```python
from build123d import *
from build123d.topology import SkipClean

# Parameters (mm, degrees)
BOSS_EXTRUDE1_START   = -10
BOSS_EXTRUDE1_DEPTH   = 40
SKETCH1_W             = 30
SKETCH1_H             = 10
BOSS_EXTRUDE1_2_DEPTH = 40
EXTRUDE_THIN1_DEPTH   = 60
BOSS_EXTRUDE2_DEPTH   = 30
BOSS_EXTRUDE3_START   = -10
BOSS_EXTRUDE3_DEPTH   = 10
FILLET2_R             = 10
BOSS_EXTRUDE4_DEPTH   = 5
CUT_EXTRUDE1_DEPTH    = 124.693168817
BOSS_EXTRUDE6_DEPTH   = 10


with BuildPart() as part:
    # Sketch1 → Boss-Extrude1 (new body)
    with BuildSketch(Plane.XY.offset(BOSS_EXTRUDE1_START)):
        with BuildLine():
            Line((60, 10), (38.729833462, 10))
            ThreePointArc((38.729833462, 10), (39.681187851, 5.040171699), (40, 0))
            Line((40, 0), (60, 0))
            Line((60, 0), (60, 10))
        make_face()
    extrude(amount=-BOSS_EXTRUDE1_DEPTH)



with BuildPart() as body_2:
    # Sketch1 → Boss-Extrude1 2 (new body)
    with BuildSketch(Plane.XY.offset(BOSS_EXTRUDE1_START)):
        with Locations((-45, 5)):
            Rectangle(SKETCH1_W, SKETCH1_H)
    extrude(amount=-BOSS_EXTRUDE1_2_DEPTH)


with BuildPart() as part_1:
    add(part.part)

    add(body_2.part)  # Extrude-Thin1 merges body 2
    # Sketch1<3> → Extrude-Thin1 (add)
    with BuildSketch(Plane.XY):
        with BuildLine():
            ThreePointArc((30, 0), (0, 30), (-30, 0))
            Line((-30, 0), (-40, 0))
            ThreePointArc((-40, 0), (0, 40), (40, 0))
            Line((40, 0), (30, 0))
        make_face()
    extrude(amount=-EXTRUDE_THIN1_DEPTH)



with BuildPart() as body_2_2:
    # Sketch2 → Boss-Extrude2 (new body)
    with BuildSketch(Plane(origin=(0, 0, -60), x_dir=(-1, 0, 0), z_dir=(0, 0, -1))):
        with BuildLine():
            ThreePointArc((-25, 100), (-17.67766953, 82.32233047), (0, 75))
            Line((0, 75), (0, 85))
            ThreePointArc((0, 85), (-10.606601718, 89.393398282), (-15, 100))
            Line((-15, 100), (-25, 100))
        make_face()
        with BuildLine():
            Line((0, 85), (0, 75))
            ThreePointArc((0, 75), (17.67766953, 82.32233047), (25, 100))
            Line((25, 100), (15, 100))
            ThreePointArc((15, 100), (10.606601718, 89.393398282), (0, 85))
        make_face()
    extrude(amount=-BOSS_EXTRUDE2_DEPTH)


with BuildPart() as part_2:
    add(part_1.part)

    add(body_2_2.part)  # Boss-Extrude3 merges body 2 2
    # Sketch2<5> → Boss-Extrude3 (add)
    with BuildSketch(Plane(origin=(0, 0, -60), x_dir=(-1, 0, 0), z_dir=(0, 0, -1)).offset(BOSS_EXTRUDE3_START)):
        with BuildLine():
            ThreePointArc((-38.239608802, 11.73594132), (-23.775642443, 32.167045659), (0, 40))
            Line((0, 40), (0, 75))
            ThreePointArc((0, 75), (-17.67766953, 82.32233047), (-25, 100))
            Line((-25, 100), (-38.239608802, 11.73594132))
        make_face()
        with BuildLine():
            Line((0, 75), (0, 40))
            ThreePointArc((0, 40), (23.775642443, 32.167045659), (38.239608802, 11.73594132))
            Line((38.239608802, 11.73594132), (25, 100))
            ThreePointArc((25, 100), (17.67766953, 82.32233047), (0, 75))
        make_face()
    extrude(amount=BOSS_EXTRUDE3_DEPTH)

    # Fillet2
    fillet2_edges = [part_2.edges().sort_by_distance(p)[0] for p in [
        (39.681187851, 5.040171699, -50),
        (-39.681187851, 5.040171699, -50),
        (-39.681187851, 5.040171699, -10),
        (39.681187851, 5.040171699, -10),
    ]]
    fillet(fillet2_edges, radius=FILLET2_R - 0.0001)  # a hair under: the kernel refuses the full size

    # Sketch3 → Boss-Extrude4 (add, symmetric)
    with BuildSketch(Plane(origin=(0, 0, 0), x_dir=(0, 0, -1), z_dir=(1, 0, 0))):
        Polygon((30, 75), (0, 40), (0, 37.743013402), (50.362835489, 37.743013402), (50.362835489, 76.354795309), (30, 76.354795309), align=None)
    extrude(amount=BOSS_EXTRUDE4_DEPTH, both=True)

    # Sketch4 → Cut-Extrude1 (cut, through all)
    with BuildSketch(Plane(origin=(0, 10, 0), x_dir=(1, 0, 0), z_dir=(0, 1, 0))):
        with BuildLine():
            Line((60, 22), (60, 38))
            ThreePointArc((60, 38), (52, 30), (60, 22))
        make_face()
        with BuildLine():
            ThreePointArc((68, 30), (65.656854249, 35.656854249), (60, 38))
            Line((60, 38), (60, 22))
            ThreePointArc((60, 22), (65.656854249, 24.343145751), (68, 30))
        make_face()
    cut_extrude1 = extrude(amount=-CUT_EXTRUDE1_DEPTH, mode=Mode.SUBTRACT)

    # Sketch4<7> → Boss-Extrude6 (add)
    with SkipClean():  # the faces are left unmerged after this step: merging them gives an invalid solid
        with BuildSketch(Plane(origin=(0, 10, 0), x_dir=(1, 0, 0), z_dir=(0, 1, 0))):
            with BuildLine():
                ThreePointArc((60, 10), (80, 30), (60, 50))
                Line((60, 50), (60, 38))
                ThreePointArc((60, 38), (65.656854249, 35.656854249), (68, 30))
                ThreePointArc((68, 30), (65.656854249, 24.343145751), (60, 22))
                Line((60, 22), (60, 10))
            make_face()
        boss_extrude6 = extrude(amount=-BOSS_EXTRUDE6_DEPTH)

    # Mirror1: Cut-Extrude1, Boss-Extrude6 across plane
    with SkipClean():  # the faces are left unmerged after this step: merging them gives an invalid solid
        add(cut_extrude1.mirror(Plane(origin=(0, 0, 0), x_dir=(0, 0, 1), z_dir=(1, 0, 0))), mode=Mode.SUBTRACT)
        add(boss_extrude6.mirror(Plane(origin=(0, 0, 0), x_dir=(0, 0, 1), z_dir=(1, 0, 0))))


solid = part_2.part
```
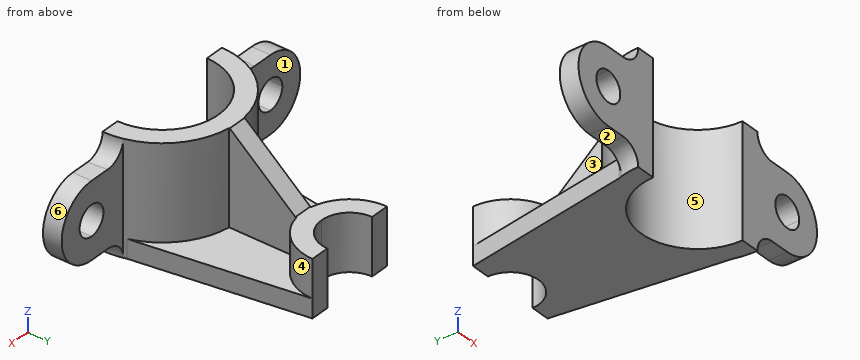
Here's how the part is built. I have some questions about the finished solid (model axes, mm). Face numbers are marked on the shaded views. A direction names the side the tool comes from. Coordinates: 2 decimals unless noted, no trailing zeros. Order: outer loops, then holes, each group sorted by start corner. A loop starts at its lowest first (then second) coordinate and runs counter-clockwise, first axis right, second up. Notation, with made-up numbers: (64.5, -7) - (108.5, -7) arc R32 ccw to (108.5, 25) - close; hole circle Ø3 at (36.5, 43). An arc over 180 degrees is marked (long way). One line per question, with ' | ' between items. Start each with the question number.
1. I'm going to push flat-ended pins straight in: pin 1 Ø5 at (y, z) = (77.5, -49) entering from +X; pin 2 Ø2 at (x, z) = (27, -24) entering from +Y; pin 3 Ø1 at (y, z) = (86.5, -35.5) entering from -X. Where does each tip first touch, or does it pass through?
2. If we section it at B-B (y = 53.5): Write out the boundary of the cut face in (x, z) (3 decimals), and give its area (3 significant figures).
3. If we section it at A-A (z = -24): Write out the boundary of the cut face in (x, y).
4. Which directions (+Z, -Z, +X, -X, +Y, -Y) give clear straight access to the entire face, cutting with the end or side of a thin tool? Please do the marked faces 1, 2 and 3.
5. Please list where these lines run through material, in increasing order: line 1 along Y through (x, z) = (-70, -25); line 2 along Z through (x, y) = (-18.5, 92.5); line 3 along X through (y, z) = (9, -33). Write a range as [from, to].
6. If we section it at D-D (x = -20.5): Write out the boundary of the cut face in (y, z), and give its area (3 significant figures).
7. If we section it at C-C (x = 28): Write out the boundary of the cut face in (y, z), and give its area (3 significant figures).
8. If we mould it in two halves opening along Y, with no side actions, what happens to the marked faces 4, 5 and 6? For each: released by +Y, released by -Y, zero draft, split by the parting line, or undercut.
Model answer:
1) pin 1: stops at x = 28.72 | pin 2: stops at y = 30.4 | pin 3: stops at x = -21.35
2) outline: (-31.975, -60) - (31.975, -60) - (31.975, -50) - (5, -50) - (5, -11.571) - (-5, -11.571) - (-5, -50) - (-31.975, -50) - close | area: 1,020 mm²
3) outline: (-79.08, 0) - (-65.29, 0) - (-65.29, 10) - (-79.08, 10) - close; (-54.71, 0) - (-30, 0) arc R30 cw to (30, 0) - (54.71, 0) - (54.71, 10) - (38.73, 10) arc R40 ccw to (5, 39.69) - (5, 68) - (-5, 68) - (-5, 39.69) arc R40 ccw to (-38.73, 10) - (-54.71, 10) - close; (65.29, 0) - (79.08, 0) - (79.08, 10) - (65.29, 10) - close
4) face 1: +Z, -Z, -X, +Y | face 2: -Z, -X, +Y, -Y | face 3: +Z, -X
5) line 1: y = [0, 10] | line 2: z = [-60, -30] | line 3: x = [-79.77, -67.42], [-52.58, -28.62], [28.62, 52.58], [67.42, 79.77]
6) outline: (21.9, -60) - (100, -60) - (100, -30) - (85.69, -30) - (85.69, -50) - (34.35, -50) - (34.35, 0) - (21.9, 0) - close | area: 1,690 mm²
7) outline: (10.77, -60) - (80, -60) - (80, -50) - (28.57, -50) - (28.57, 0) - (10.77, 0) - close | area: 1,580 mm²
8) face 4: undercut | face 5: released by -Y | face 6: zero draft
